Can you work these out from the drawing? Everything is in mm from the part's minimum corner. A direction names the side the tool comes from. Coordinates: 2 decimals unless noted, no trailing zeros. Write each loop counter-clockwise with the first axis right and the second up, starting at its lowest first coordinate (ties: lowest second). Pieces come first, ordered by that corner, then holes. Notation, with made-up numbers: (-21, 87) -> (32, 87) arc R35 ccw to (32, 125) -> close; hole circle Ø7 at (53.5, 53). An arc over 180 degrees is marked (long way). Use a Markdown table: item, result. Add a question column.
Item 1: On a 3-axis mill with a long thin cutter (end or side, diameter ignored), from which of +Z, -Z, +X, -X, +Y, -Y can I reach the whole of each face in a straight line? I mean the marked faces 4 and 5. Say none if no direction works.
Item 2: Imagine slicing it at A-A, the plane z = 22.5. Write out the boundary of the cut face in (x, y).
Item 3: Imagine slicing it at D-D, the plane x = 0.65. Write out the boundary of the cut face in (y, z), and give its area (3 significant figures).
Item 4: If I drill on line 1 along Y through (x, z) = (2.95, 22.5); line 2 along Z through (x, y) = (3.8, 9.5) (1 decimal); line 3 along Z through (x, y) = (0.6, 36.5) (1 decimal), over which ranges is the centre line in solid material (lowest first)? Write a range as from..to.
Item 5: Will these pins go through, and if not, where does the flat tip stop? pin 1 Ø3 at (x, z) = (1, 31.5) entering from -Y; pin 2 Ø2.5 at (y, z) = (35.76, 9.24) entering from +X; pin 3 Ø3 at (x, z) = (2.5, 9.5) entering from -Y; pin 4 Ø4 at (y, z) = (9.5, 8.5) entering from +X.
Item 6: If we mould it in two halves opening along Y, with no side actions, what happens to the marked faces 1, 2 and 3? For each: pulls with the +Y half, pulls with the -Y half, needs draft (parallel to the pull), parting line crosses it, or undercut.
Item 7: Imagine slicing it at C-C, the plane z = 33.5. Write out the boundary of the cut face in (x, y), and give its area (3 significant figures).
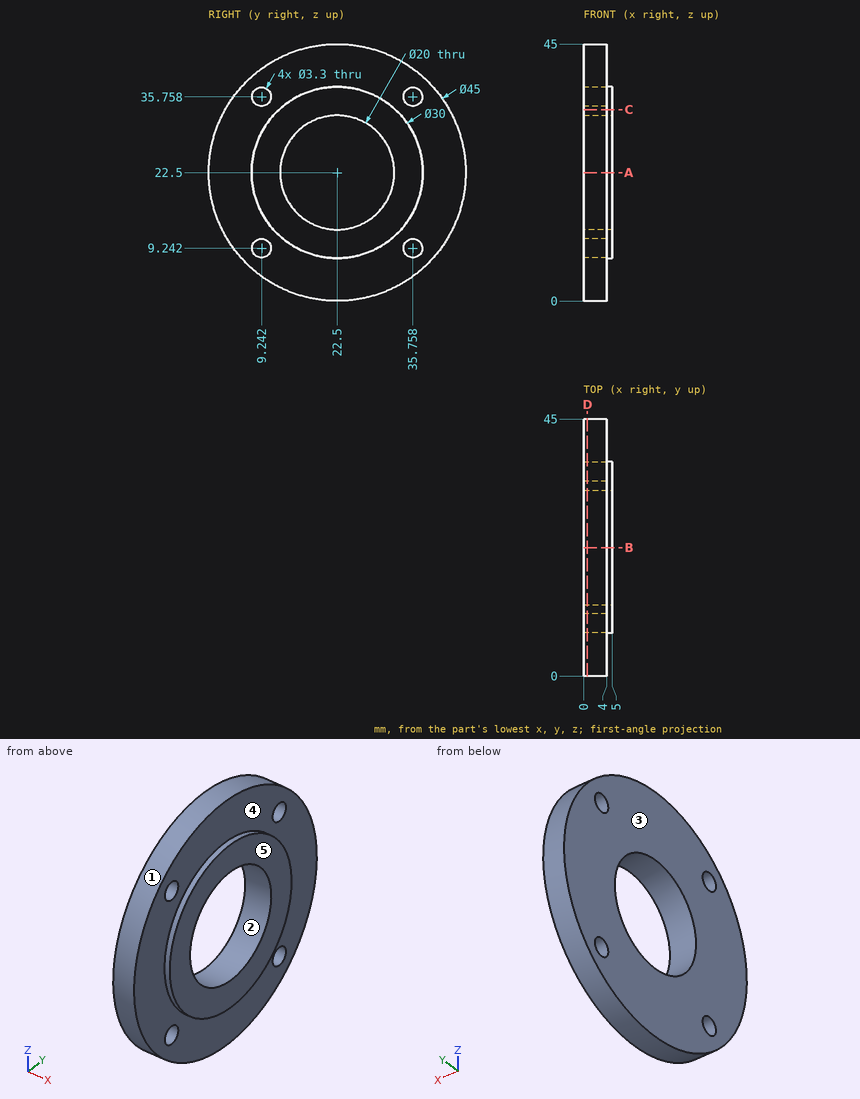
Ans:
| question | item | result |
|---|---|---|
| 1 | face 4 | +X |
| 1 | face 5 | +Z, -Z, +X, +Y, -Y |
| 2 | outline | (0, 0) -> (4, 0) -> (4, 7.5) -> (5, 7.5) -> (5, 12.5) -> (0, 12.5) -> close; (0, 32.5) -> (5, 32.5) -> (5, 37.5) -> (4, 37.5) -> (4, 45) -> (0, 45) -> close |
| 3 | outline | circle Ø45 at (22.5, 22.5); hole circle Ø3.3 at (9.24, 9.24); hole circle Ø3.3 at (9.24, 35.76); hole circle Ø20 at (22.5, 22.5); hole circle Ø3.3 at (35.76, 9.24); hole circle Ø3.3 at (35.76, 35.76) |
| 3 | area | 1,240 mm^2 |
| 4 | line 1 | y = 0..12.5, 32.5..45 |
| 4 | line 2 | z = 4.1..7.6, 10.9..34.1, 37.4..40.9 |
| 4 | line 3 | z = 4.9..7.8, 10.7..34.3, 37.2..40.1 |
| 5 | pin 1 | stops at y = 1.29 |
| 5 | pin 2 | passes through |
| 5 | pin 3 | stops at y = 3.16 |
| 5 | pin 4 | stops at x = 4 |
| 6 | face 1 | parting line crosses it |
| 6 | face 2 | undercut |
| 6 | face 3 | needs draft |
| 7 | outline | (0, 2.87) -> (4, 2.87) -> (4, 12.3) -> (5, 12.3) -> (5, 32.7) -> (4, 32.7) -> (4, 42.13) -> (0, 42.13) -> close |
| 7 | area | 177 mm^2 |
